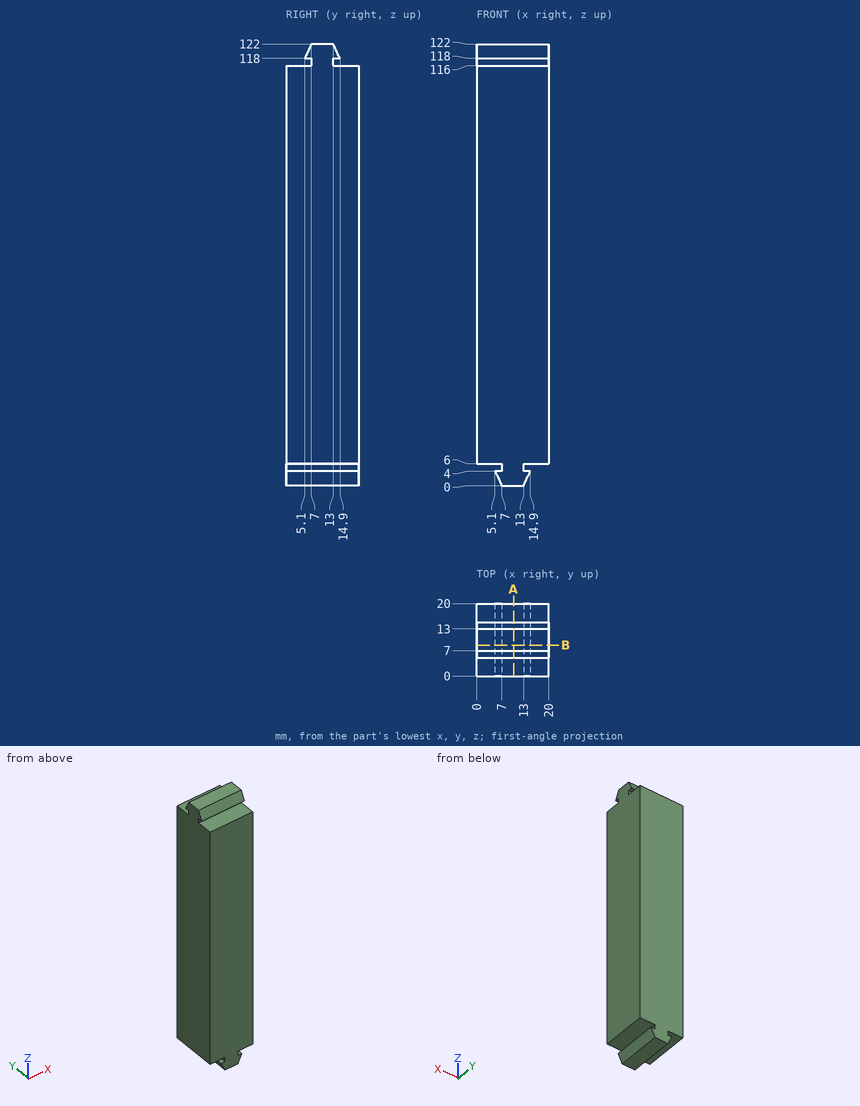
Study the drawing (mm; zero at the part's minimum x, y, z) and answer. Give positions to 0.01 mm unless a question says otherwise; leave off trailing zeros. Write each loop counter-clockwise with the first axis right and the second up, starting at its lowest first coordinate (ties: lowest second). Pieces come first, ordered by that corner, then holes. Notation, with made-up numbers: (-35.5, 66.5) -> (-22.5, 66.5) arc R18 ccw to (-22.5, 101.5) -> close; hole circle Ø9 at (13.5, -19.5). An arc over 180 degrees is marked (long way). Write item = value, one per line. Start each with the question number.
1) Each of these flat-tipped pins is pushed along its axis until it touches: pin 1 (2 mm diameter, centred on x = 11.5, y = 5, fed in from +Z); pin 2 (1.5 mm diameter, centred on x = 4.5, y = 14.5, fed in from +Z); pin 3 (2 mm diameter, centred on x = 11, y = 18, fed in from +Z). Where does it stop, or does it pass through?
2) Straight lines are drawn through the part: line 1 along Z through (x, y) = (18.5, 2); line 2 along Z through (x, y) = (6.5, 9); line 3 along Z through (x, y) = (9, 14.25). For each, find the intervals that lie inside material, in ascending order.
3) The part is cut by section A-A, the plane x = 10.25. Determine the outline of the cut face in (y, z).
4) The part is cut by section B-B, the plane y = 8.5. Determine the outline of the cut face in (x, z), and give its area (3 significant figures).
Solutions:
q1.pin_1 = 119.89
q1.pin_2 = 120.42
q1.pin_3 = 116
q2.line_1 = 6 to 116
q2.line_2 = 1.05 to 4, 6 to 122
q2.line_3 = 0 to 116, 118 to 119.37
q3.outline = (0, 0) -> (20, 0) -> (20, 116) -> (13, 116) -> (13, 118) -> (14.9, 118) -> (13, 122) -> (7, 122) -> (5.1, 118) -> (7, 118) -> (7, 116) -> (0, 116) -> close
q4.outline = (0, 6) -> (7, 6) -> (7, 4) -> (5.1, 4) -> (7, 0) -> (13, 0) -> (14.9, 4) -> (13, 4) -> (13, 6) -> (20, 6) -> (20, 122) -> (0, 122) -> close
q4.area = 2,360 mm²
